Design review of the part built by this model. Coordinates are the model's own, in mm. A direction names the side the tool comes from. Coordinates: 2 decimals unless noted, no trailing zeros. Loops run counter-clockwise (first coordinate to the right, second up) from the corner with the lowest first, then second, coordinate; pieces in that order, holes last. Notation, with made-up numbers: (-12, 28.5) - (40, 28.5) arc R23 cw to (40, 62.5) - close; hole circle Ø11 at (23, 31.25). An arc over 180 degrees is marked (long way). Return JSON: item names as keys, results as strings. Group by question number.
from build123d import *

# Parameters (mm, degrees)
SKETCH1_R           = 1.5
BOSS_EXTRUDE1_DEPTH = 2
SKETCH2_R           = 0.75
BOSS_EXTRUDE2_DEPTH = 5.3
FILLET1_R           = 0.5


with BuildPart() as part:
    # Sketch1 → Boss-Extrude1 (new body)
    with BuildSketch(Plane.XY):
        Circle(SKETCH1_R)
    extrude(amount=BOSS_EXTRUDE1_DEPTH)

    # Sketch2 → Boss-Extrude2 (add)
    with BuildSketch(Plane.XY.offset(2)):
        Circle(SKETCH2_R)
    extrude(amount=BOSS_EXTRUDE2_DEPTH)

    # Fillet1
    fillet1_edges = [part.edges().sort_by_distance(p)[0] for p in [
        (-0.75, 0, 7.3),
    ]]
    fillet(fillet1_edges, radius=FILLET1_R)


solid = part.part
Item 1: For P1, Ø1, axis at x = 0, z = 4, coming from the +Y side; P2, Ø1, axis at x = -1, y = 1, coming from the +Z side, all flat-tipped, find the tip position at first contact; note any pin that passes through.
Item 2: Add section B-B (z = 1.75). State the section outline as (x, y) points.
Item 3: For faces 1 (the face through (0, 0, 0)), 2 (the face through (-0.75, 0.03, 4.37)), list the 3-axis set-ups (+Z, -Z, +X, -X, +Y, -Y) from which the entire face can be reached by the end or side of a thin tool; tool diameter is ignored.
Item 4: Add section A-A (z = 3.5). State the section outline as (x, y) points.
Item 5: To check wall thickness, follow line 1 (Z direction, x = -0.15, y = 0.9); line 2 (Z direction, x = 0.6, y = -0.2); line 3 (X direction, y = -0.3, z = 2.25). State the ranges of each line that lie inside material, in increasing order. Write a range as from..to.
Answers below:
{
 "1": {"P1": "stops at y = 0.75", "P2": "stops at z = 2"},
 "2": {"outline": "circle Ø3 at (0, 0)"},
 "3": {"face 1": "-Z, +X, -X, +Y, -Y", "face 2": "+Z"},
 "4": {"outline": "circle Ø1.5 at (0, 0)"},
 "5": {"line 1": "z = 0..2", "line 2": "z = 0..7.12", "line 3": "x = -0.69..0.69"}
}
